from build123d import *

# Parameters (mm, degrees)
SKETCH1_W                  = 50.8
SKETCH1_H                  = 74.6125
BOSS_EXTRUDE1_DEPTH        = 57.15
SKETCH2_W                  = 31.75
SKETCH2_H                  = 61.9125
CUT_EXTRUDE1_DEPTH         = 47.625
FILLET1_R                  = 6.35
CUT_EXTRUDE2_REACH         = 76.612
SKETCH3_R                  = 15.875
F_6_32_TAPPED_HOLE1_D      = 2.7051
F_6_32_TAPPED_HOLE1_DEPTH  = 7.62
F_6_32_TAPPED_HOLE1_TIP    = 0.81269403
SKETCH8_W                  = 9.525
SKETCH8_H                  = 57.15
BOSS_EXTRUDE2_DEPTH        = 10
M5_CLEARANCE_HOLE1_D       = 5.3
M5_CLEARANCE_HOLE1_DEPTH   = 9.525
CUT_EXTRUDE3_REACH         = 62.8
SKETCH11_R                 = 13.208
F_10_32_TAPPED_HOLE2_D     = 4.0386
F_10_32_TAPPED_HOLE2_DEPTH = 4.826
F_10_32_TAPPED_HOLE2_TIP   = 1.213317848
F_2_56_TAPPED_HOLE1_D      = 1.778
F_2_56_TAPPED_HOLE1_DEPTH  = 6.604
F_2_56_TAPPED_HOLE1_TIP    = 0.53416509
F_6_32_TAPPED_HOLE2_D      = 2.7051
F_6_32_TAPPED_HOLE2_DEPTH  = 9.0424
F_6_32_TAPPED_HOLE2_TIP    = 0.81269403
CUT_EXTRUDE6_REACH         = 76.613


with BuildPart() as part:
    # Sketch1 → Boss-Extrude1 (new body)
    with BuildSketch(Plane(origin=(0, 0, 0), x_dir=(1, 0, 0), z_dir=(0, 1, 0))):
        Rectangle(SKETCH1_W, SKETCH1_H)
    extrude(amount=BOSS_EXTRUDE1_DEPTH)

    # Sketch2 → Cut-Extrude1 (cut)
    with BuildSketch(Plane(origin=(0, 57.15, 0), x_dir=(1, 0, 0), z_dir=(0, 1, 0))):
        Rectangle(SKETCH2_W, SKETCH2_H)
    extrude(amount=-CUT_EXTRUDE1_DEPTH, mode=Mode.SUBTRACT)

    # Fillet1
    fillet1_edges = [part.edges().sort_by_distance(p)[0] for p in [
        (-15.875, 33.3375, -30.95625),
        (-15.875, 33.3375, 30.95625),
        (15.875, 33.3375, 30.95625),
        (15.875, 33.3375, -30.95625),
    ]]
    fillet(fillet1_edges, radius=FILLET1_R)

    # Sketch3 → Cut-Extrude2 (cut, up to next)
    with BuildSketch(Plane(origin=(0, 0, -37.30625), x_dir=(-1, 0, 0), z_dir=(0, 0, -1)), mode=Mode.PRIVATE) as cut_extrude2_sk1:
        with Locations((0, 32.825)):
            Circle(SKETCH3_R)
    cut_extrude2_tool1 = extrude(cut_extrude2_sk1.sketch, amount=-CUT_EXTRUDE2_REACH, mode=Mode.PRIVATE) & part.part
    add(cut_extrude2_tool1.solids().sort_by_distance((0, 32.825, -37.30625))[0], mode=Mode.SUBTRACT)

    # #6-32 Tapped Hole1
    with Locations(Plane(origin=(0, 57.15, 0), x_dir=(-1, 0, 0), z_dir=(0, 1, 0))):
        with Locations((20.6375, -32.54375), (-20.6375, -32.54375), (20.6375, 32.54375), (-20.6375, 32.54375)):
            Hole(F_6_32_TAPPED_HOLE1_D / 2, depth=F_6_32_TAPPED_HOLE1_DEPTH)
            with Locations((0, 0, -(F_6_32_TAPPED_HOLE1_DEPTH + F_6_32_TAPPED_HOLE1_TIP / 2))):  # 118° drill point
                Cone(0, F_6_32_TAPPED_HOLE1_D / 2, F_6_32_TAPPED_HOLE1_TIP, mode=Mode.SUBTRACT)

    # Sketch8 → Boss-Extrude2 (add)
    with BuildSketch(Plane.ZY.offset(25.4)):
        with Locations((-32.54375, 28.575)):
            Rectangle(SKETCH8_W, SKETCH8_H)
    boss_extrude2 = extrude(amount=BOSS_EXTRUDE2_DEPTH)

    # Mirror1: Boss-Extrude2 across plane
    add(boss_extrude2.mirror(Plane(origin=(0, 0, 0), x_dir=(0, 0, 1), z_dir=(1, 0, 0))))

    # M5 Clearance Hole1
    with Locations(Plane(origin=(0, 0, -37.30625), x_dir=(-1, 0, 0), z_dir=(0, 0, -1))):
        with Locations((30, 12.827), (30, 52.827), (-30, 52.827), (-30, 12.827)):
            Hole(M5_CLEARANCE_HOLE1_D / 2, depth=M5_CLEARANCE_HOLE1_DEPTH)

    # Sketch11 → Cut-Extrude3 (cut, up to next)
    with BuildSketch(Plane.ZY.offset(25.4), mode=Mode.PRIVATE) as cut_extrude3_sk1:
        with Locations((7.20725, 28.575)):
            Circle(SKETCH11_R)
    cut_extrude3_tool1 = extrude(cut_extrude3_sk1.sketch, amount=-CUT_EXTRUDE3_REACH, mode=Mode.PRIVATE) & part.part
    add(cut_extrude3_tool1.solids().sort_by_distance((-25.4, 28.575, 7.20725))[0], mode=Mode.SUBTRACT)

    # #10-32 Tapped Hole2
    with Locations(Plane.ZY.offset(25.4)):
        with Locations((-16.79575, 28.575), (-4.79425, 49.362207767), (19.20875, 49.362207767), (31.21025, 28.575), (19.20875, 7.787792233), (-4.79425, 7.787792233)):
            Hole(F_10_32_TAPPED_HOLE2_D / 2, depth=F_10_32_TAPPED_HOLE2_DEPTH)
            with Locations((0, 0, -(F_10_32_TAPPED_HOLE2_DEPTH + F_10_32_TAPPED_HOLE2_TIP / 2))):  # 118° drill point
                Cone(0, F_10_32_TAPPED_HOLE2_D / 2, F_10_32_TAPPED_HOLE2_TIP, mode=Mode.SUBTRACT)

    # #2-56 Tapped Hole1
    with Locations(Plane(origin=(0, 9.525, 0), x_dir=(-1, 0, 0), z_dir=(0, 1, 0))):
        with Locations((13, -12.163354521), (13, -25.163354521), (-13, -25.163354521), (-13, -12.163354521), (5.6515, 4.74375), (-5.6515, 4.74375)):
            Hole(F_2_56_TAPPED_HOLE1_D / 2, depth=F_2_56_TAPPED_HOLE1_DEPTH)
            with Locations((0, 0, -(F_2_56_TAPPED_HOLE1_DEPTH + F_2_56_TAPPED_HOLE1_TIP / 2))):  # 118° drill point
                Cone(0, F_2_56_TAPPED_HOLE1_D / 2, F_2_56_TAPPED_HOLE1_TIP, mode=Mode.SUBTRACT)

    # #6-32 Tapped Hole2
    with Locations(Plane.XY.offset(37.30625)):
        with Locations((20.50625, 48.141034847), (20.50625, 6.866034847), (-20.76875, 48.141034847), (-20.76875, 6.866034847)):
            Hole(F_6_32_TAPPED_HOLE2_D / 2, depth=F_6_32_TAPPED_HOLE2_DEPTH)
            with Locations((0, 0, -(F_6_32_TAPPED_HOLE2_DEPTH + F_6_32_TAPPED_HOLE2_TIP / 2))):  # 118° drill point
                Cone(0, F_6_32_TAPPED_HOLE2_D / 2, F_6_32_TAPPED_HOLE2_TIP, mode=Mode.SUBTRACT)

    # Sketch24 → Cut-Extrude6 (cut, up to next)
    with BuildSketch(Plane.XY.offset(37.30625), mode=Mode.PRIVATE) as cut_extrude6_sk1:
        with BuildLine():
            Line((-4.7625, 11.628534847), (4.7625, 11.628534847))
            ThreePointArc((4.7625, 11.628534847), (8.130096045, 13.023438801), (9.525, 16.391034847))
            Line((9.525, 16.391034847), (9.525, 38.616034847))
            ThreePointArc((9.525, 38.616034847), (8.130096045, 41.983630892), (4.7625, 43.378534847))
            Line((4.7625, 43.378534847), (-4.7625, 43.378534847))
            ThreePointArc((-4.7625, 43.378534847), (-8.130096045, 41.983630892), (-9.525, 38.616034847))
            Line((-9.525, 38.616034847), (-9.525, 16.391034847))
            ThreePointArc((-9.525, 16.391034847), (-8.130096045, 13.023438801), (-4.7625, 11.628534847))
        make_face()
    cut_extrude6_tool1 = extrude(cut_extrude6_sk1.sketch, amount=-CUT_EXTRUDE6_REACH, mode=Mode.PRIVATE) & part.part
    add(cut_extrude6_tool1.solids().sort_by_distance((0, 27.503535, 37.30625))[0], mode=Mode.SUBTRACT)


solid = part.part
Part model, mm, in its own coordinate system. A direction names the side the tool comes from. Coordinates: 2 decimals unless noted, no trailing zeros. Order: outer loops, then holes, each group sorted by start corner. A loop starts at its lowest first (then second) coordinate and runs counter-clockwise, first axis right, second up.
(1) Pin check, flat tips, straight feed: pin 1 Ø5 at (y, z) = (12.5, -12) entering from +X; pin 2 Ø2 at (x, y) = (-20.77, 6.87) entering from +Z; pin 3 Ø1.6 at (x, z) = (13, -25.16) entering from +Y. Stop position of each tip, or through.
Check sheet entries:
pin 1: stops at x = 25.4
pin 2: stops at z = 28.05
pin 3: stops at y = 2.87
(2) Slice it at A-A, the plane x = -30. Write the cut outline in (y, z).
Check sheet entries:
outline: (0, -37.31) - (10.18, -37.31) - (10.18, -27.78) - (0, -27.78) - close; (15.48, -37.31) - (50.18, -37.31) - (50.18, -27.78) - (15.48, -27.78) - close; (55.48, -37.31) - (57.15, -37.31) - (57.15, -27.78) - (55.48, -27.78) - close
(3) Slice it at D-D, the plane x = 0. Write the cut outline in (y, z) (3 decimals).
Check sheet entries:
outline: (0, -37.306) - (16.95, -37.306) - (16.95, -30.956) - (9.525, -30.956) - (9.525, 30.956) - (11.629, 30.956) - (11.629, 37.306) - (0, 37.306) - close; (43.379, 30.956) - (57.15, 30.956) - (57.15, 37.306) - (43.379, 37.306) - close; (48.7, -37.306) - (57.15, -37.306) - (57.15, -30.956) - (48.7, -30.956) - close
(4) Tool access for faces 4 (the face through (15.86, 33.52, -32.46)), 5 (the face through (21.365, 53.287, 33.684)), 6 (the face through (-22.953, 28.664, 33.228)), 7 (the face through (-22.02, 6.35, 32.72)): list every direction of +Z, -Z, +X, -X, +Y, -Y with a clear straight run to the whole face (end or side of a thin tool).
Check sheet entries:
face 4: -Z
face 5: +Y
face 6: -X
face 7: +Z
(5) Slice it at C-C, the plane z = 7. Write the cut outline in (x, y) (3 decimals), and give its area (3 significant figures).
Check sheet entries:
outline: (-25.4, 0) - (25.4, 0) - (25.4, 57.15) - (15.875, 57.15) - (15.875, 9.525) - (-15.875, 9.525) - (-15.875, 15.369) - (-25.4, 15.369) - close; (-25.4, 41.781) - (-15.875, 41.781) - (-15.875, 57.15) - (-25.4, 57.15) - close
area: 1,140 mm2
(6) Pull direction X, two halves, no side cores. Call faces 1 (the face through (8.167, 41.946, 34.176)), 2 (the face through (25.4, 28, 5)), 3 (the face through (-25.4, 15, 5)): pulls with the +X half, pulls with the -X half, needs draft (parallel to the pull), parting line crosses it, or undercut.
Check sheet entries:
face 1: undercut
face 2: pulls with the +X half
face 3: pulls with the -X half
(7) Slice it at B-B, the plane y = 22.5. Write the cut outline in (x, z) (3 decimals).
Check sheet entries:
outline: (-35.4, -37.306) - (-12.059, -37.306) - (-12.059, -30.429) arc R6.35 cw to (-15.875, -24.606) - (-15.875, -4.521) - (-25.4, -4.521) - (-25.4, -27.781) - (-35.4, -27.781) - close; (-25.4, 18.935) - (-15.875, 18.935) - (-15.875, 24.606) arc R6.35 cw to (-9.525, 30.956) - (-9.525, 37.306) - (-25.4, 37.306) - close; (9.525, 30.956) arc R6.35 cw to (15.875, 24.606) - (15.875, -24.606) arc R6.35 cw to (12.059, -30.429) - (12.059, -37.306) - (35.4, -37.306) - (35.4, -27.781) - (25.4, -27.781) - (25.4, 37.306) - (9.525, 37.306) - close
(8) Probe L1, parallel to Z at x = 13, y = 4; L2, parallel to X at y = 19, z = -20.5 (3 decimals); L3, parallel to X at y = 51, z = -29. List the from-to ranges inside material, lowest first.
Check sheet entries:
L1: z = -37.31 to -26.05, -24.27 to -13.05, -11.27 to 37.31
L2: x = -25.4 to -15.875, 15.875 to 25.4
L3: x = -35.4 to -31.92, -28.08 to -14.11, 14.11 to 28.08, 31.92 to 35.4
